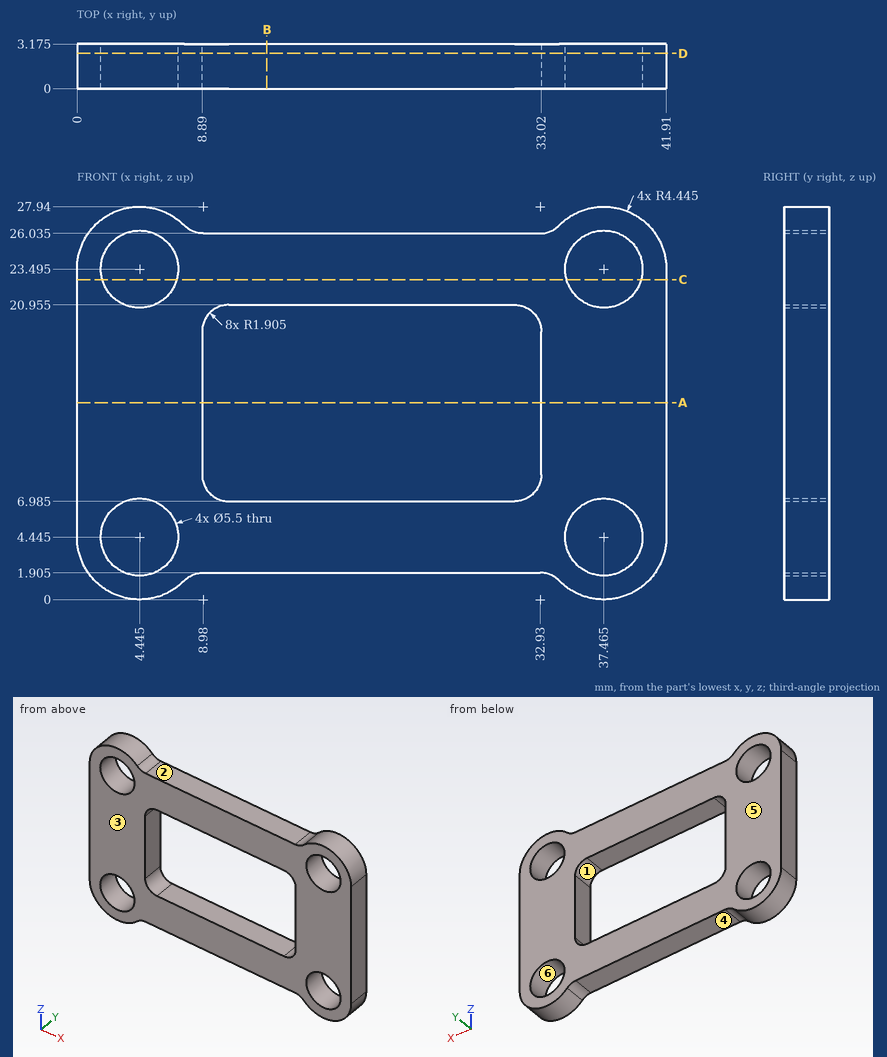
Input: dimensioned drawing with shaded views. Units: mm. Origin: part minimum x, y, z. A direction names the side the tool comes from. Coordinates: 2 decimals unless noted, no trailing zeros. Loops run counter-clockwise (first coordinate to the right, second up) from the corner with the lowest first, then second, coordinate; pieces in that order, holes last. Notation, with made-up numbers: M 7,19.5 L 52,19.5 A21 cw 52,24.5 Z; hole C 9.5,-8 d7. An arc over 180 degrees is marked long. One line per item, written item: value. Start each with the question number.
1) Material intervals for L1, parallel to Z at x = 12.5, y = 2 (3 decimals); L2, parallel to X at y = 1.55, z = 18.5; L3, parallel to X at y = 0.35, z = 2 (1 decimal), sorted ascending. Write a range as from..to.
2) Cut plane B-B (x = 13.5). Return loops of the section in (y, z) (3 decimals).
3) Reachability of the marked faces 1, 2, 3 and 4 from +Z, -Z, +X, -X, +Y, -Y: full face, straight path, thin tool, end or side. Return the list, or none.
4) Cut plane D-D (y = 2.5). Count the separate pieces of the cut face and the enclosed holes in it, then the cut area to 3 significant figures.
5) Cut plane C-C (z = 22.75). Return loops of the section in (x, y) (1 decimal).
6) Draft query along X for the marked faces 5 and 6. Return one class per face: released by +X, released by -X, zero draft, split by the parting line, or undercut.
7) Cut plane A-A (z = 14). Return loops of the section in (x, y) (3 decimals).
8) Pin query (flat end, axial travel): P1, Ø1.6, axis at x = 18, y = 1, coming from the +Z side (3 decimals); P2, Ø1.5, axis at x = 7, y = 1, coming from the -Z side; P3, Ø1, axis at x = 17, y = 2, coming from the -Z side (3 decimals). Return the tip coordinate at first contact, or that it passes through.
Evaluation:
1. L1: 1.905..6.985, 20.955..26.035
1. L2: 0..8.89, 33.02..41.91
1. L3: 0.7..3.2, 5.7..36.2, 38.7..41.2
2. outline: M 0,1.905 L 3.175,1.905 L 3.175,6.985 L 0,6.985 Z; M 0,20.955 L 3.175,20.955 L 3.175,26.035 L 0,26.035 Z
3. face 1: +Y, -Y
3. face 2: +Z, +Y, -Y
3. face 3: +Z, -Z, +X, -X, -Y
3. face 4: -Z, +Y, -Y
4. separate pieces: 1
4. enclosed holes: 5
4. area: 619 mm^2
5. outline: M 0,0 L 1.8,0 L 1.8,3.2 L 0,3.2 Z; M 7.1,0 L 34.8,0 L 34.8,3.2 L 7.1,3.2 Z; M 40.1,0 L 41.9,0 L 41.9,3.2 L 40.1,3.2 Z
6. face 5: zero draft
6. face 6: undercut
7. outline: M 0,0 L 8.89,0 L 8.89,3.175 L 0,3.175 Z; M 33.02,0 L 41.91,0 L 41.91,3.175 L 33.02,3.175 Z
8. P1: z = 26.035
8. P2: z = 0.38
8. P3: z = 1.905
